```python
from build123d import *

# Parameters (mm, degrees)
RESSALTO_EXTRUS_O1_DEPTH = 3.1
ESBO_O3_R                = 2.25
ESBO_O2_R                = 0.45
ESBO_O4_R                = 0.2
CORTE_EXTRUS_O1_DEPTH    = 6.2


with BuildPart() as part:
    # Esboço1 → Ressalto-extrusão1 (new body)
    with BuildSketch(Plane.XY):
        Polygon((-3.637009085, 1.6), (-1.67401817, 5), (-3.637009085, 8.4), (-7.562990915, 8.4), (-9.52598183, 5), (-7.562990915, 1.6), align=None)
    extrude(amount=RESSALTO_EXTRUS_O1_DEPTH)

    # Esboço3 → Loft3 section 0
    with BuildSketch(Plane.XY.offset(3.1)):
        with Locations((-5.6, 5)):
            Circle(ESBO_O3_R)
    # Esboço2 → Loft3 section 1
    with BuildSketch(Plane.XY.offset(5.2)):
        with Locations((-5.6, 5)):
            Circle(ESBO_O2_R)
    loft()

    # Esboço4 → Corte-extrusão1 (cut, through all)
    with BuildSketch(Plane.XY.offset(5.2)):
        with Locations((-5.6, 5)):
            Circle(ESBO_O4_R)
    extrude(amount=-CORTE_EXTRUS_O1_DEPTH, mode=Mode.SUBTRACT)


solid = part.part
```
Check sheet for the modelled part. Datum: model origin and axes. Units: mm. A direction names the side the tool comes from. Round coordinates to 2 decimals unless told otherwise and drop trailing zeros. Loops run counter-clockwise (first coordinate to the right, second up) from the corner with the lowest first, then second, coordinate; pieces in that order, holes last. Notation, with made-up numbers: (-17, 79) -> (26, 79) arc R21 cw to (26, 86) -> close; hole circle Ø5 at (-21, -20). An arc over 180 degrees is marked (long way). Answer in a Markdown table with one row per item.
Q1. Thickness scan on L1, parallel to Y at x = -5.6, z = 2.95; L2, parallel to Z at x = -3.25, y = 5.75; L3, parallel to Z at x = -5.5, y = 6. Record the ranges inside material, lowest first.
Data:
| item | result |
|---|---|
| L1 | y = 1.6 to 4.8, 5.2 to 8.4 |
| L2 | z = 0 to 3.1 |
| L3 | z = 0 to 4.55 |
Q2. Set-up check for faces 1 (the face through (-4, 7, 3.1)), 2 (the face through (-8.558, 3.324, 1.528)): record each of +Z, -Z, +X, -X, +Y, -Y from which the full face is reachable in a straight line by a thin tool's end or side.
Data:
| item | result |
|---|---|
| face 1 | +Z |
| face 2 | +Z, -Z, -X, -Y |
Q3. Sectioned sample at C-C on z = 3.45. Enter the section's corners in (x, y).
Data:
| item | result |
|---|---|
| outline | circle Ø3.9 at (-5.6, 5); hole circle Ø0.4 at (-5.6, 5) |
Q4. Sectioned sample at A-A on z = 2.5. Enter the section's corners in (x, y).
Data:
| item | result |
|---|---|
| outline | (-9.53, 5) -> (-7.56, 1.6) -> (-3.64, 1.6) -> (-1.67, 5) -> (-3.64, 8.4) -> (-7.56, 8.4) -> close; hole circle Ø0.4 at (-5.6, 5) |
Q5. Go/stop test with flat-tipped pins: P1, Ø4, axis at x = -4, y = 7.5, coming from the +Z side; P2, Ø2, axis at y = 4.5, z = 4, coming from the +X side; P3, Ø1, axis at y = 4, z = 3.5, coming from the +X side. Record where each tip stops, or that it passes through.
Data:
| item | result |
|---|---|
| P1 | stops at z = 4.6 |
| P2 | stops at x = -1.71 |
| P3 | stops at x = -2.08 |
Q6. Sectioned sample at D-D on x = -2.25. Enter the section's corners in (y, z), then the cut area to 3 significant figures.
Data:
| item | result |
|---|---|
| outline | (4, 0) -> (6, 0) -> (6, 3.1) -> (4, 3.1) -> close |
| area | 6.19 mm^2 |
Q7. Sectioned sample at B-B on x = -5.6. Enter the section's corners in (y, z), then the cut area to 3 significant figures.
Data:
| item | result |
|---|---|
| outline | (1.6, 0) -> (4.8, 0) -> (4.8, 5.2) -> (4.55, 5.2) -> (2.75, 3.1) -> (1.6, 3.1) -> close; (5.2, 0) -> (8.4, 0) -> (8.4, 3.1) -> (7.25, 3.1) -> (5.45, 5.2) -> (5.2, 5.2) -> close |
| area | 24.7 mm^2 |
